```python
from build123d import *

# Parameters (mm, degrees)
SKETCH_W      = 54
SKETCH_H      = 76
SKETCH_R      = 3.5
EXTRUDE_DEPTH = 10
FILLET_R      = 3


with BuildPart() as part:
    # Sketch → Extrude (new body)
    with BuildSketch(Plane.XY):
        Rectangle(SKETCH_W, SKETCH_H)
        with Locations((-20.5, 31)):
            Circle(SKETCH_R, mode=Mode.SUBTRACT)
        with Locations((20.5, 31)):
            Circle(SKETCH_R, mode=Mode.SUBTRACT)
        with Locations((-20.5, -22)):
            Circle(SKETCH_R, mode=Mode.SUBTRACT)
        with Locations((20.5, -22)):
            Circle(SKETCH_R, mode=Mode.SUBTRACT)
    extrude(amount=EXTRUDE_DEPTH)

    # Fillet
    fillet_edges = [part.edges().sort_by_distance(p)[0] for p in [
        (-27, 38, 5),
        (27, 38, 5),
        (27, -38, 5),
        (-27, -38, 5),
    ]]
    fillet(fillet_edges, radius=FILLET_R)


solid = part.part
```
Check sheet for the modelled part. Datum: model origin and axes. Units: mm. Coordinates: 2 decimals unless noted, no trailing zeros. Loops run counter-clockwise (first coordinate to the right, second up) from the corner with the lowest first, then second, coordinate; pieces in that order, holes last.
1) Material ranges on probe 1 along Y at (x, z) = (-20.5, 5.75); probe 2 along X at (y, z) = (34, 2); probe 3 along X at (y, z) = (-19.5, 3.5), recorded low to high.
2) Sectioned sample at A-A (y = -22). Record the boundary of the cut face in (x, z), and give its area (3 significant figures).
3) Sectioned sample at C-C (z = 8.25). Record the boundary of the cut face in (x, y), and give its area (3 significant figures).
4) Release check for a two-part mould opening along Y. For faces 1 (the face through (0, -38, 5)), 2 (the face through (26.1, 37.14, 5.07)), 3 (the face through (22.38, -19.05, 4.93)) record: released by +Y, released by -Y, zero draft, split by the parting line, or undercut.
5) Sectioned sample at B-B (x = -20.5). Record the boundary of the cut face in (y, z), and give its area (3 significant figures).
Check sheet entries:
1. probe 1: y = -38 to -25.5, -18.5 to 27.5, 34.5 to 38
1. probe 2: x = -27 to -22.3, -18.7 to 18.7, 22.3 to 27
1. probe 3: x = -27 to -22.95, -18.05 to 18.05, 22.95 to 27
2. outline: (-27, 0) - (-24, 0) - (-24, 10) - (-27, 10) - close; (-17, 0) - (17, 0) - (17, 10) - (-17, 10) - close; (24, 0) - (27, 0) - (27, 10) - (24, 10) - close
2. area: 400 mm2
3. outline: (-27, -35) arc R3 ccw to (-24, -38) - (24, -38) arc R3 ccw to (27, -35) - (27, 35) arc R3 ccw to (24, 38) - (-24, 38) arc R3 ccw to (-27, 35) - close; hole circle Ø7 at (-20.5, -22); hole circle Ø7 at (-20.5, 31); hole circle Ø7 at (20.5, -22); hole circle Ø7 at (20.5, 31)
3. area: 3,940 mm2
4. face 1: released by -Y
4. face 2: released by +Y
4. face 3: undercut
5. outline: (-38, 0) - (-25.5, 0) - (-25.5, 10) - (-38, 10) - close; (-18.5, 0) - (27.5, 0) - (27.5, 10) - (-18.5, 10) - close; (34.5, 0) - (38, 0) - (38, 10) - (34.5, 10) - close
5. area: 620 mm2
